Verification items for the finished model (mm, model axes). Face numbers are marked on the shaded views. A direction names the side the tool comes from. Round coordinates to 2 decimals unless told otherwise and drop trailing zeros. Write each loop counter-clockwise with the first axis right and the second up, starting at its lowest first coordinate (ties: lowest second). Pieces come first, ordered by that corner, then holes. Notation, with made-up numbers: (64.5, 66) - (111.5, 66) arc R17 cw to (111.5, 81) - close; hole circle Ø11 at (61, 21.5). An arc over 180 degrees is marked (long way). Answer as a JSON object with one key per item and string values. Group by question number.
1) Go/stop test with flat-tipped pins: pin 1 Ø1 at (y, z) = (-11.5, 1) entering from +X; pin 2 Ø3.5 at (x, y) = (6.13, 23.02) entering from +Z; pin 3 Ø1.5 at (x, z) = (-6, 1.5) entering from +Y; pin 4 Ø6 at (x, y) = (-10, -8) entering from +Z. Record where each tip stops, or that it passes through.
2) Section check A-A (x = -10). Enter the section's corners in (y, z), then the cut area to 3 significant figures.
3) Section check C-C (z = 5.5). Enter the section's corners in (x, y).
4) Section check D-D (z = 1.25). Enter the section's corners in (x, y), then the cut area to 3 significant figures.
5) Mould release check, pull along X, two halves, no side actions. Record for the marked faces 4, 5 and 6: +X half, -X half, draft (parallel to the pull), parting line (faces both ways), or undercut.
6) Section check B-B (y = 2.5). Enter the section's corners in (x, z), then the cut area to 3 significant figures.
7) Set-up check for the marked faces 1, 2 and 3: record each of +Z, -Z, +X, -X, +Y, -Y from which the full face is reachable in a straight line by a thin tool's end or side.
8) Thickness scan on line 1 (X direction, y = 3, z = 1.5); line 2 (Z direction, x = -16.5, y = 11); line 3 (X direction, y = 2, z = 4.25). Record the ranges inside material, lowest first.
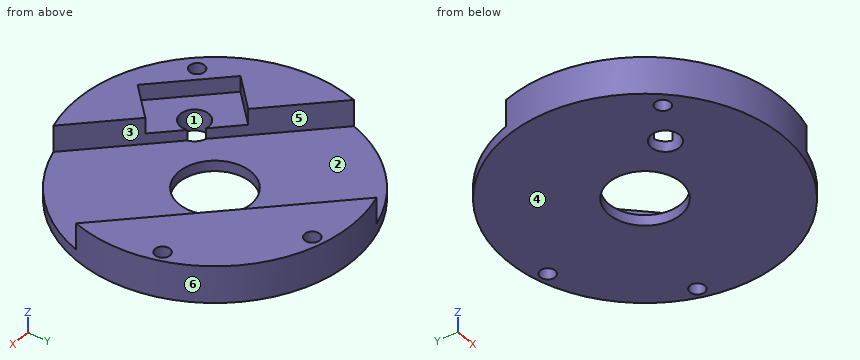
Autodesk Inventor part; units mm, degrees
ref_plane "YZ Plane" through (0, 0, 0) normal (1, 0, 0) x (0, 1, 0)
ref_plane "XZ Plane" through (0, 0, 0) normal (0, 1, 0) x (-1, 0, 0)
ref_plane "XY Plane" through (0, 0, 0) normal (0, 0, 1) x (1, 0, 0)
ref_plane "Work Plane1" through (0, 0, 0) normal (0, 0, 1) x (1, 0, 0)
sketch "Sketch1" plane through (0, 0, 0) normal (0, 0, 1) x (1, 0, 0)
  circle A0 centre (0, 0) radius 25.9979
  circle A1 centre (-9.4998, -11.0022) radius 2.6601
  circle A2 centre (0.0001, -0.0022) radius 3.8801
  circle A3 centre (0.0001, -0.0022) radius 6.7754
  point P0 (0, 0)
extrude "Extrusion1" add sketch "Sketch1" along normal blind 7 contours A0
sketch "Sketch2" plane through (0, 0, 7) normal (0, 0, 1) x (1, 0, 0)
  line L0 (32.4435, -15.1193) -> (-15.1193, 32.4435)
  line L1 (-15.1193, 32.4435) -> (-32.4435, 15.1193)
  line L2 (-32.4435, 15.1193) -> (15.1193, -32.4435)
  line L3 (15.1193, -32.4435) -> (32.4435, -15.1193)
  line L4 (32.4435, -15.1193) -> (-32.4435, 15.1193) construction
  line L5 (-15.1193, 32.4435) -> (15.1193, -32.4435) construction
  line L6 (32.4435, -15.1193) -> (99.7074, -15.1193) construction
  point P0 (0, 0)
  dimension "d2" = 135
  dimension "d3" = 24.5
extrude "Extrusion2" cut sketch "Sketch2" against normal blind 5
sketch "Sketch3" plane through (0, 0, 7) normal (0, 0, 1) x (1, 0, 0)
  line L0 (-7.7936, -20.2561) -> (-2.9652, -15.4277)
  line L1 (-18.7537, -9.2959) -> (-13.9253, -4.4675)
  line L2 (-13.5111, -3.9119) -> (-2.4095, -15.0135)
  line L3 (-2.4095, -15.0135) -> (-8.2078, -20.8117)
  line L4 (-8.2078, -20.8117) -> (-19.3094, -9.7102)
  line L5 (-19.3094, -9.7102) -> (-13.5111, -3.9119)
  line L6 (-8.9176, -8.4066) -> (-24.8767, 7.5526)
  line L7 (-13.4617, -3.8624) -> (-2.4095, -15.0135)
  line L8 (-2.4095, -15.0135) -> (-0.3384, -12.9607)
  line L9 (-0.3384, -12.9607) -> (-11.3905, -1.8096)
  line L10 (-11.3905, -1.8096) -> (-13.4617, -3.8624)
  line L11 (-13.4617, -3.8624) -> (-13.5111, -3.9119)
  line L12 (-8.9176, -8.4066) -> (-24.8767, 7.5526)
  line L13 (-13.9253, -4.4675) -> (-2.9652, -15.4277)
  line L14 (-7.7936, -20.2561) -> (-18.7537, -9.2959)
  point P0 (0, 0)
  dimension "d6" = 0.1
extrude "Extrusion3" cut sketch "Sketch3" against normal blind 3 contours L14 L1 L13 L0 | L11 L7 L2 | L2 L3 L4 L5 | L7 L10 L9 L8
sketch "Skizze4" plane through (0, 0, 7) normal (0, 0, 1) x (1, 0, 0)
  spline S0 degree 2 poles (24.1427, 2.2394) (24.731, 1.8489) (25.3785, 0.5587) (25.3785, -0.3311) knots 0 0 0 1 2 2 2 construction
  spline S1 degree 2 poles (25.3785, -0.3311) (25.3785, -1.1665) (24.7013, -2.5111) (24.1328, -2.8867) knots 0 0 0 1 2 2 2 construction
  spline S2 degree 2 poles (24.1328, -2.8867) (23.6682, -3.1784) (22.7141, -3.3761) (21.9726, -3.3761) knots 0 0 0 1 2 2 2 construction
  line L0 (21.9726, -3.3761) -> (20.5687, -3.3761) construction
  line L1 (20.5687, -3.3761) -> (20.5687, 2.7239) construction
  line L2 (20.5687, 2.7239) -> (21.9578, 2.7239) construction
  spline S3 degree 2 poles (21.9578, 2.7239) (22.8179, 2.7239) (23.7967, 2.4668) (24.1427, 2.2394) knots 0 0 0 1 2 2 2 construction
  spline S4 degree 2 poles (19.1896, -2.9312) (18.8979, -3.1982) (18.1564, -3.4849) (17.5978, -3.4849) knots 0 0 0 1 2 2 2 construction
  spline S5 degree 2 poles (17.5978, -3.4849) (16.9354, -3.4849) (16.0061, -3.2081) (15.5958, -3.0103) knots 0 0 0 1 2 2 2 construction
  line L3 (15.5958, -3.0103) -> (15.5958, -1.992) construction
  line L4 (15.5958, -1.992) -> (15.6551, -1.992) construction
  spline S6 degree 2 poles (15.6551, -1.992) (16.0555, -2.3677) (17.0689, -2.7829) (17.5385, -2.7829) knots 0 0 0 1 2 2 2 construction
  spline S7 degree 2 poles (17.5385, -2.7829) (18.2108, -2.7829) (18.8979, -2.2243) (18.8979, -1.7646) knots 0 0 0 1 2 2 2 construction
  spline S8 degree 2 poles (18.8979, -1.7646) (18.8979, -1.3988) (18.5371, -0.944) (18.1465, -0.8303) knots 0 0 0 1 2 2 2 construction
  spline S9 degree 2 poles (18.1465, -0.8303) (17.8648, -0.7513) (17.3952, -0.6425) (17.0442, -0.5535) knots 0 0 0 1 2 2 2 construction
  spline S10 degree 2 poles (17.0442, -0.5535) (16.7278, -0.4695) (16.2285, -0.2174) (16.0358, -0.0147) knots 0 0 0 1 2 2 2 construction
  spline S11 degree 2 poles (16.0358, -0.0147) (15.8479, 0.188) (15.6403, 0.7317) (15.6403, 1.0876) knots 0 0 0 1 2 2 2 construction
  spline S12 degree 2 poles (15.6403, 1.0876) (15.6403, 1.8291) (16.797, 2.8326) (17.6918, 2.8326) knots 0 0 0 1 2 2 2 construction
  spline S13 degree 2 poles (17.6918, 2.8326) (18.2059, 2.8326) (19.1154, 2.6299) (19.5059, 2.4372) knots 0 0 0 1 2 2 2 construction
  line L5 (19.5059, 2.4372) -> (19.5059, 1.4683) construction
  line L6 (19.5059, 1.4683) -> (19.4466, 1.4683) construction
  spline S14 degree 2 poles (19.4466, 1.4683) (19.155, 1.7352) (18.2454, 2.1307) (17.7461, 2.1307) knots 0 0 0 1 2 2 2 construction
  spline S15 degree 2 poles (17.7461, 2.1307) (17.1826, 2.1307) (16.4856, 1.6017) (16.4856, 1.1717) knots 0 0 0 1 2 2 2 construction
  spline S16 degree 2 poles (16.4856, 1.1717) (16.4856, 0.7861) (16.8959, 0.3264) (17.2815, 0.2226) knots 0 0 0 1 2 2 2 construction
  spline S17 degree 2 poles (17.2815, 0.2226) (17.5385, 0.1534) (18.285, -0.0246) (18.5321, -0.0987) knots 0 0 0 1 2 2 2 construction
  spline S18 degree 2 poles (18.5321, -0.0987) (19.1599, -0.2915) (19.7432, -1.0676) (19.7432, -1.6361) knots 0 0 0 1 2 2 2 construction
  spline S19 degree 2 poles (19.7432, -1.6361) (19.7432, -1.997) (19.4516, -2.689) (19.1896, -2.9312) knots 0 0 0 1 2 2 2 construction
  circle A0 centre (-9.9998, 17.4978) radius 1.3999 construction
  circle A1 centre (10.0001, 17.4979) radius 1.4 construction
  circle A2 centre (10.0001, -17.5021) radius 1.4 construction
  circle A3 centre (-9.9998, -17.5021) radius 1.4001 construction
  arc A4 (-25.1198, 6.6998) -> (-24.1417, 5.4917) centre (-24.1417, 6.4917) ccw construction
  line L7 (-24.1417, 5.4917) -> (-17.7002, 5.4917) construction
  arc A5 (-15.7002, 3.4917) -> (-17.7002, 5.4917) centre (-17.7002, 3.4917) ccw construction
  line L8 (-15.7002, 3.4917) -> (-15.7002, -4.496) construction
  arc A6 (-17.7002, -6.496) -> (-15.7002, -4.496) centre (-17.7002, -4.496) ccw construction
  line L9 (-17.7002, -6.496) -> (-23.8502, -6.496) construction
  arc A7 (-23.8502, -6.496) -> (-24.8235, -7.7254) centre (-23.8502, -7.496) ccw construction
  arc A8 (-24.8235, -7.7254) -> (-25.1198, 6.6998) centre (0, 0) ccw construction
  circle A9 centre (-9.4998, -11.0022) radius 2.6601 construction
  circle A10 centre (-16.8291, -16.0482) radius 1.4 construction
  circle A11 centre (6.1284, 23.0202) radius 1.4 construction
  circle A12 centre (22.7119, 7.1872) radius 1.4 construction
  circle A13 centre (0.0001, -0.0022) radius 6.5 construction
  point P0 (0, 0)
hole "Bohrung1" at (6.1284, 23.0202, 7) at (22.7119, 7.1872, 7) at (-16.8291, -16.0482, 7) direction (0, 0, -1) diameter 2.8 end through all
properties part number "Matchboxscope_sample_v1"
Returned:
{
 "1": {"pin 1": "x = 23.56", "pin 2": "z = 7", "pin 3": "y = 25.46", "pin 4": "z = 4"},
 "2": {"outline": "(-24, 0) - (-13.61, 0) - (-13.61, 4) - (-19.02, 4) - (-19.02, 7) - (-24, 7) - close; (-8.39, 0) - (24, 0) - (24, 2) - (-7.32, 2) - (-7.32, 4) - (-8.39, 4) - close", "area": "123 mm2"},
 "3": {"outline": "(-24.88, 7.55) arc R26 ccw to (7.55, -24.88) - (-2.36, -14.96) - (-2.41, -15.01) - (-8.21, -20.81) - (-19.31, -9.71) - (-13.51, -3.91) - (-13.46, -3.86) - close; (-7.55, 24.88) - (24.88, -7.55) arc R26 ccw to start; hole circle Ø2.8 at (-16.83, -16.05); hole circle Ø2.8 at (6.13, 23.02); hole circle Ø2.8 at (22.71, 7.19)"},
 "4": {"outline": "circle Ø52 at (0, 0); hole circle Ø2.8 at (-16.83, -16.05); hole circle Ø5.32 at (-9.5, -11); hole circle Ø13.55 at (0, 0); hole circle Ø2.8 at (6.13, 23.02); hole circle Ø2.8 at (22.71, 7.19)", "area": "1,940 mm2"},
 "5": {"face 4": "draft", "face 5": "undercut", "face 6": "parting line"},
 "6": {"outline": "(-25.88, 0) - (-6.3, 0) - (-6.3, 2) - (-19.82, 2) - (-19.82, 7) - (-25.88, 7) - close; (6.3, 0) - (25.88, 0) - (25.88, 7) - (14.82, 7) - (14.82, 2) - (6.3, 2) - close", "area": "164 mm2"},
 "7": {"face 1": "+Z, -Z", "face 2": "+Z", "face 3": "+Z, +X"},
 "8": {"line 1": "-25.82 to -6.07, 6.07 to 25.82", "line 2": "0 to 2", "line 3": "-25.92 to -19.32, 15.32 to 25.92"}
}
